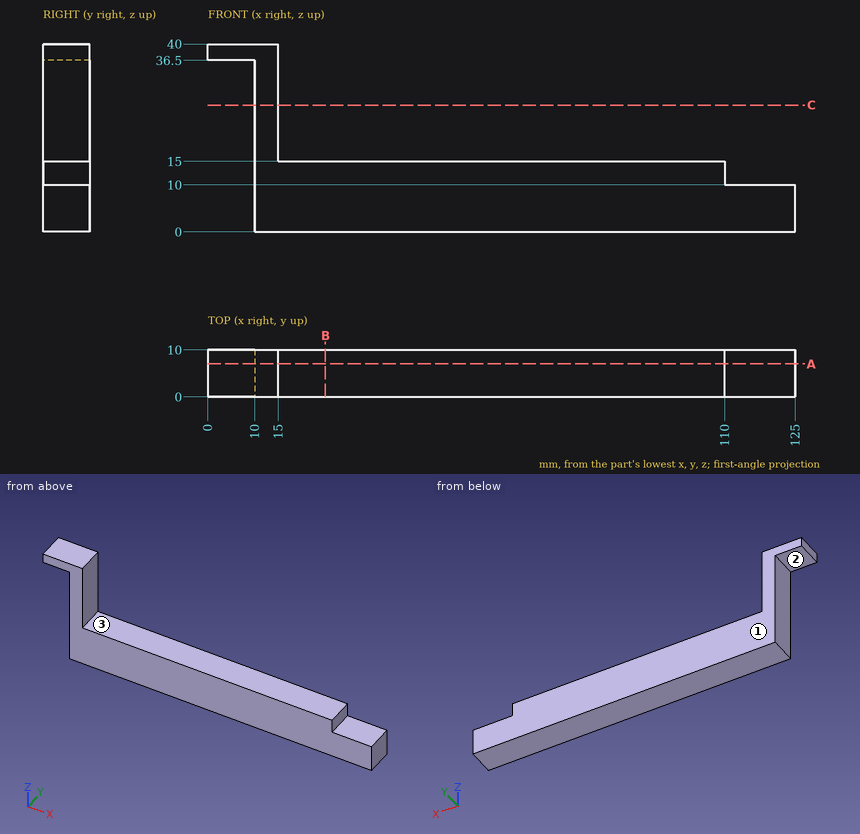
The drawing under review shows one solid part. Ordinate dimensions are in mm from its lowest x, y, z. A direction names the side the tool comes from. Give positions to 0.01 mm unless a question says otherwise; leave off trailing zeros. Order: outer loops, then holes, each group sorted by start corner. A loop starts at its lowest first (then second) coordinate and runs counter-clockwise, first axis right, second up. Notation, with made-up numbers: M 40,2 L 75,2 A18 cw 75,6 Z; hole C 20.5,-28.5 d5. An arc over 180 degrees is marked long. Answer in a Markdown table with one row per item. Add a question column.
1. Add section B-B on x = 25. State the section outline as (y, z) points.
2. For pin 1 Ø1.5 at (y, z) = (4, 20) entering from +X; pin 2 Ø3 at (x, y) = (6, 7.5) entering from -Z; pin 3 Ø2 at (x, y) = (42, 8.5) entering from +Z, all flat-tipped, find the tip position at first contact; note any pin that passes through.
3. Add section C-C on z = 27. State the section outline as (x, y) points.
4. Machinability: for the marked faces 1, 2 and 3, which of the approach directions +Z, -Z, +X, -X, +Y, -Y give a long, thin tool a straight path to every point of the face, cutting with its end or side? Answer none if there is none.
5. To check wall thickness, follow line 1 along Z through (x, y) = (84, 5); line 2 along X through (y, z) = (5.5, 26); line 3 along X through (y, z) = (3, 3). State the ranges of each line that lie inside material, in increasing order.
6. Add section A-A on y = 7. State the section outline as (x, z) points, plus the area to 3 significant figures.
The answers:
| question | item | result |
|---|---|---|
| 1 | outline | M 0,0 L 10,0 L 10,15 L 0,15 Z |
| 2 | pin 1 | x = 15 |
| 2 | pin 2 | z = 36.5 |
| 2 | pin 3 | z = 15 |
| 3 | outline | M 10,0 L 15,0 L 15,10 L 10,10 Z |
| 4 | face 1 | +Z, -Z, +X, -X, +Y |
| 4 | face 2 | -Z, -X, +Y, -Y |
| 4 | face 3 | +Z, +X, +Y, -Y |
| 5 | line 1 | 0 to 15 |
| 5 | line 2 | 10 to 15 |
| 5 | line 3 | 10 to 125 |
| 6 | outline | M 0,36.5 L 10,36.5 L 10,0 L 125,0 L 125,10 L 110,10 L 110,15 L 15,15 L 15,40 L 0,40 Z |
| 6 | area | 1,810 mm2 |
